Source: three-view drawing plus pictorial views. Frame: mm from the lowest corner of the part. Coordinates: 2 decimals unless noted, no trailing zeros. Write each loop counter-clockwise with the first axis right and the second up, starting at its lowest first coordinate (ties: lowest second). Pieces come first, ordered by that corner, then holes. Notation, with made-up numbers: (19.5, -13) - (40.5, -13) arc R23 cw to (40.5, -5) - close; hole circle Ø2 at (-3.5, -5.5). An arc over 180 degrees is marked (long way). Put each result on its own line as item: value.
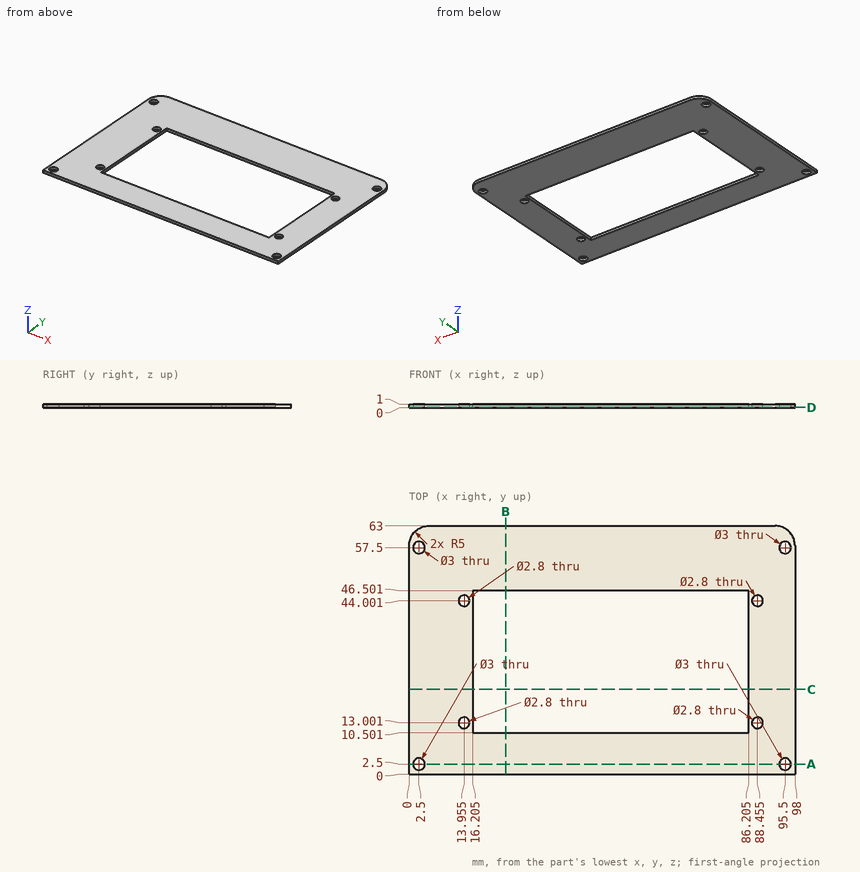
1. Ray query, probe 1 along X at (y, z) = (44, 0.8) (1 decimal); probe 2 along Y at (x, z) = (26, 0.5); probe 3 along X at (y, z) = (33, 0.8) (1 decimal). Return the intervals inside material, ascending. Write a range as from..to.
Answer below:
probe 1: x = 0..12.6, 15.4..16.2, 86.2..87.1, 89.9..98
probe 2: y = 0..10.5, 46.5..63
probe 3: x = 0..16.2, 86.2..98
2. Section query D-D (z = 0.15). Count the separate pieces of the cut face and the enclosed holes in it, then the cut area to 3 significant figures.
Answer below:
separate pieces: 1
enclosed holes: 9
area: 3,590 mm²
3. Section query B-B (x = 24.5). Return loops of the section in (y, z), then the cut area to 3 significant figures.
Answer below:
outline: (0, 0) - (10.5, 0) - (10.5, 1) - (0, 1) - close; (46.5, 0) - (63, 0) - (63, 1) - (46.5, 1) - close
area: 27.0 mm²
4. Section query A-A (y = 2.5). Return loops of the section in (x, z).
Answer below:
outline: (0, 0) - (1, 0) - (1, 1) - (0, 1) - close; (4, 0) - (94, 0) - (94, 1) - (4, 1) - close; (97, 0) - (98, 0) - (98, 1) - (97, 1) - close
5. Section query C-C (y = 21.5). Return loops of the section in (x, z) (1 decimal), then the cut area to 3 significant figures.
Answer below:
outline: (0, 0) - (16.2, 0) - (16.2, 1) - (0, 1) - close; (86.2, 0) - (98, 0) - (98, 1) - (86.2, 1) - close
area: 28.0 mm²
